Model file for the job. Use its own axes, mm. Face numbers are marked on the shaded views. Round coordinates to 2 decimals unless told otherwise and drop trailing zeros. Order: outer loops, then holes, each group sorted by start corner. A loop starts at its lowest first (then second) coordinate and runs counter-clockwise, first axis right, second up. Notation, with made-up numbers: (20.5, -15) -> (48.5, -15) arc R23 cw to (48.5, 15) -> close; hole circle Ø4 at (77, -40). An arc over 180 degrees is marked (long way). Put each result on its own line as item: value. Start each with the question number.
Q1. Pull direction Y, two halves, no side cores. Call the marked faces 1 and 2: released by +Y, released by -Y, zero draft, split by the parting line, or undercut.
Q2. Cut at C-C, the plane x = 0. List the corners of the cut face in (y, z), and give its area (3 significant figures).
Q3. Cut at B-B, the plane y = 0. List the corners of the cut face in (x, z).
Q4. Probe L1, parallel to X at y = -0.5, z = 1.5; L2, parallel to Z at x = 1.5, y = -33; L3, parallel to X at y = -44.5, z = 1.25. List the from-to ranges inside material, lowest first.
Q5. Flat gauge pins, fed straight in: P1, Ø1.8, axis at x = -64, z = 2, coming from the -Y side; P2, Ø1.5, axis at x = 49.5, z = 4.5, coming from the -Y side; P3, Ø1, axis at x = 4.5, z = 3.5, coming from the +Y side. Where does each tip first touch, or does it go through?
from build123d import *

# Parameters (mm, degrees)
BOSS_EXTRUDE1_DEPTH = 6
BOSS_EXTRUDE2_START = -1
SKETCH1_2_R         = 62.5
BOSS_EXTRUDE2_DEPTH = 1
CUT_EXTRUDE1_DEPTH  = 89.591760339
BOSS_EXTRUDE3_START = -1
BOSS_EXTRUDE3_DEPTH = 7
CHAMFER1_SIZE       = 1


with BuildPart() as part:
    # Sketch1 → Boss-Extrude1 (new body)
    with BuildSketch(Plane.XY):
        with BuildLine():
            ThreePointArc((-60.751522615, -4.25), (-60.9, 0), (-60.751522615, 4.25))
            Line((-60.751522615, 4.25), (-62.355332571, 4.25))
            ThreePointArc((-62.355332571, 4.25), (-62.5, 0), (-62.355332571, -4.25))
            Line((-62.355332571, -4.25), (-60.751522615, -4.25))
        make_face()
        with BuildLine():
            Line((-62.355332571, 4.25), (-60.751522615, 4.25))
            ThreePointArc((-60.751522615, 4.25), (2.126296401, 60.862869334), (60.9, 0))
            ThreePointArc((60.9, 0), (2.126296401, -60.862869334), (-60.751522615, -4.25))
            Line((-60.751522615, -4.25), (-62.355332571, -4.25))
            ThreePointArc((-62.355332571, -4.25), (-62.295612153, -5.050416467), (-62.225617715, -5.85))
            ThreePointArc((-62.225617715, -5.85), (2.928215567, -62.431366745), (62.5, 0))
            ThreePointArc((62.5, 0), (2.928215567, 62.431366745), (-62.225617715, 5.85))
            ThreePointArc((-62.225617715, 5.85), (-62.295612153, 5.050416467), (-62.355332571, 4.25))
        make_face()
    extrude(amount=BOSS_EXTRUDE1_DEPTH)

    # Sketch1<2> → Boss-Extrude2 (add)
    with BuildSketch(Plane.XY.offset(BOSS_EXTRUDE2_START)):
        Circle(SKETCH1_2_R)
    extrude(amount=BOSS_EXTRUDE2_DEPTH)

    # Sketch1<4> → Cut-Extrude1 (cut, symmetric)
    with BuildSketch(Plane.XY):
        with BuildLine():
            ThreePointArc((-60.751522615, -4.25), (-60.9, 0), (-60.751522615, 4.25))
            Line((-60.751522615, 4.25), (-62.355332571, 4.25))
            ThreePointArc((-62.355332571, 4.25), (-62.5, 0), (-62.355332571, -4.25))
            Line((-62.355332571, -4.25), (-60.751522615, -4.25))
        make_face()
    cut_extrude1 = extrude(amount=CUT_EXTRUDE1_DEPTH, both=True, mode=Mode.SUBTRACT)

    # Sketch1<5> → Boss-Extrude3 (add)
    with BuildSketch(Plane.XY.offset(BOSS_EXTRUDE3_START)):
        with BuildLine():
            Line((-63.1627417, 4.25), (-62.355332571, 4.25))
            ThreePointArc((-62.355332571, 4.25), (-62.295612153, 5.050416467), (-62.225617715, 5.85))
            Line((-62.225617715, 5.85), (-64.7627417, 5.85))
            Line((-64.7627417, 5.85), (-64.7627417, -5.85))
            Line((-64.7627417, -5.85), (-62.225617715, -5.85))
            ThreePointArc((-62.225617715, -5.85), (-62.295612153, -5.050416467), (-62.355332571, -4.25))
            Line((-62.355332571, -4.25), (-63.1627417, -4.25))
            Line((-63.1627417, -4.25), (-63.1627417, 4.25))
        make_face()
    boss_extrude3 = extrude(amount=BOSS_EXTRUDE3_DEPTH)

    # Mirror1: Cut-Extrude1, Boss-Extrude3 across plane
    add(cut_extrude1.mirror(Plane(origin=(0, 0, 0), x_dir=(0, 0, 1), z_dir=(1, 0, 0))), mode=Mode.SUBTRACT)
    add(boss_extrude3.mirror(Plane(origin=(0, 0, 0), x_dir=(0, 0, 1), z_dir=(1, 0, 0))))

    # Chamfer1
    chamfer1_edges = [part.edges().sort_by_distance(p)[0] for p in [
        (0, -60.9, 0),
        (0, -62.5, -1),
        (0, 60.9, 0),
        (0, 62.5, -1),
    ]]
    chamfer(chamfer1_edges, length=CHAMFER1_SIZE - 0.0001)  # a hair under: the kernel refuses the full size


solid = part.part
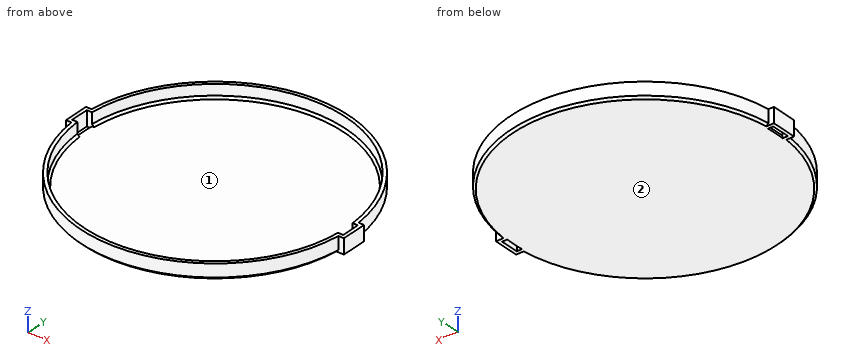
Ans:
1. face 1: undercut
1. face 2: zero draft
2. outline: (-62.5, 0) -> (-61.5, -1) -> (61.5, -1) -> (62.5, 0) -> (62.5, 6) -> (60.9, 6) -> (60.9, 1) -> (59.9, 0) -> (-59.9, 0) -> (-60.9, 1) -> (-60.9, 6) -> (-62.5, 6) -> close
2. area: 144 mm^2
3. outline: (-64.76, -1) -> (-63.16, -1) -> (-63.16, 6) -> (-64.76, 6) -> close; (-60.9, -1) -> (60.9, -1) -> (60.9, 0) -> (-60.9, 0) -> close; (63.16, -1) -> (64.76, -1) -> (64.76, 6) -> (63.16, 6) -> close
4. L1: x = -64.76 to -63.16, 63.16 to 64.76
4. L2: z = -1 to 0
4. L3: x = -43.89 to -41.58, 41.58 to 43.89
5. P1: stops at y = -5.85
5. P2: stops at y = -39.11
5. P3: stops at y = 62.37
